The model under review builds one solid part; all positions refer to its coordinate system, in mm. Coordinates: 2 decimals unless noted, no trailing zeros. Loops run counter-clockwise (first coordinate to the right, second up) from the corner with the lowest first, then second, coordinate; pieces in that order, holes last. Notation, with made-up numbers: M 9.5,-13 L 52.5,-13 A20 cw 52.5,-9 Z; hole C 16,-19 d9. An arc over 180 degrees is marked long. Write item = value, one per line. Start each with the question number.
Q1. Wall thickness on probe 1 along X at (y, z) = (7.75, -249.5); probe 2 along X at (y, z) = (4, -135); probe 3 along Z at (x, y) = (-130.5, 10): over which ranges is each line inside the solid? List them lowest first.
Q2. We need section C-C on x = -31. Give the boundary of the cut face in (y, z).
Q3. We need section A-A on y = 3. Give the boundary of the cut face in (x, z), and give its area (3 significant figures).
Q4. We need section B-B on z = -168.5. Give the boundary of the cut face in (x, y), and give its area (3 significant figures).
Q5. Clearance check with flat-ended pins moving along their axes: pin 1 Ø6 at (x, y) = (-115, 9) entering from -Z; pin 2 Ø1 at (y, z) = (7, -255.5) entering from -X; pin 3 Ø5 at (x, y) = (-89, 5.5) entering from -Z. State where each tip first meets the part, or that it passes through.
from build123d import *

# Parameters (mm, degrees)
BOSS_EXTRUDE1_DEPTH = 12.7


with BuildPart() as part:
    # Sketch1 → Boss-Extrude1 (new body)
    with BuildSketch(Plane(origin=(0, 0, 0), x_dir=(1, 0, 0), z_dir=(0, 1, 0))):
        with BuildLine():
            Line((-2.671745921, 8.296474175), (-60.783183135, 188.74777921))
            Line((-60.783183135, 188.74777921), (-61.817176572, 191.958600936))
            ThreePointArc((-61.817176572, 191.958600936), (-62.442896831, 193.322917601), (-63.371363054, 194.502254821))
            Line((-63.371363054, 194.502254821), (-65.756579877, 196.887471644))
            Line((-65.756579877, 196.887471644), (-165.560118982, 296.691010749))
            ThreePointArc((-165.560118982, 296.691010749), (-170.050247042, 298.550882688), (-174.540375103, 296.691010749))
            Line((-174.540375103, 296.691010749), (-181.72458, 289.506805852))
            ThreePointArc((-181.72458, 289.506805852), (-183.584451939, 285.016677791), (-181.72458, 280.526549731))
            Line((-181.72458, 280.526549731), (-85.480125087, 184.282094819))
            ThreePointArc((-85.480125087, 184.282094819), (-84.551658864, 183.102757598), (-83.925938605, 181.738440933))
            Line((-83.925938605, 181.738440933), (-26.818084588, 4.403525825))
            ThreePointArc((-26.818084588, 4.403525825), (-24.512913596, 1.217621847), (-20.773770045, 0))
            Line((-20.773770045, 0), (-8.716060463, 0))
            ThreePointArc((-8.716060463, 0), (-3.58368231, 2.610856449), (-2.671745921, 8.296474175))
        make_face()
    extrude(amount=BOSS_EXTRUDE1_DEPTH)


solid = part.part
Returned:
q1.probe_1 = -150.7 to -118.37
q1.probe_2 = -68.87 to -43.47
q1.probe_3 = -261.63 to -229.3
q2.outline = M 0,-96.26 L 12.7,-96.26 L 12.7,-17.39 L 0,-17.39 Z
q3.outline = M -181.72,-289.51 L -174.54,-296.69 A6.35 ccw -165.56,-296.69 L -63.37,-194.5 A6.35 ccw -61.82,-191.96 L -2.67,-8.3 A6.35 ccw -8.72,0 L -20.77,0 A6.35 ccw -26.82,-4.4 L -83.93,-181.74 A6.35 cw -85.48,-184.28 L -181.72,-280.53 A6.35 ccw Z
q3.area = 8,130 mm^2
q4.outline = M -79.66,0 L -54.26,0 L -54.26,12.7 L -79.66,12.7 Z
q4.area = 323 mm^2
q5.pin_1 = -249.13
q5.pin_2 = -157.2
q5.pin_3 = -222.63
